The figure shows three views and two pictorial views of one solid part (mm, origin at its lowest corner). Answer the questions. A direction names the side the tool comes from. Give positions to 0.01 mm unless a question says otherwise; leave off trailing zeros. Loops run counter-clockwise (first coordinate to the right, second up) from the corner with the lowest first, then second, coordinate; pieces in that order, holes last. Notation, with made-up numbers: M 26.25,-0.5 L 69.25,-0.5 A20 cw 69.25,28.5 Z; hole C 27.5,-7.75 d9. An arc over 180 degrees is marked long. Write item = value, one per line. Start each with the question number.
1. Section B-B on z = 114.3 is taken. Determine the outline of the cut face in (x, y) (1 decimal).
2. Flat-ended cylindrical pins translate along their axes: pin 1 Ø10 at (x, y) = (28, 11.5) entering from +Z; pin 2 Ø10.5 at (y, z) = (12.5, 109.5) entering from +X (3 decimals); pin 3 Ø17.5 at (x, z) = (20.5, 104.5) entering from +Y (3 decimals). Find the tip coordinate at first contact, or state that the pin passes through.
3. Section D-D on x = 24 is taken. Determine the outline of the cut face in (y, z) (1 decimal).
4. Consider L1, parallel to Z at x = 2, y = 19; L2, parallel to Y at x = 2.45, z = 38.1; L3, parallel to Y at x = 23, z = 145 (1 decimal). Determine where each line is inside the solid, lowest interval first. Write a range as [from, to].
5. Section C-C on z = 57 is taken. Determine the outline of the cut face in (x, y) (1 decimal).
6. For the marked faces 1 and 2, determine the directions among +Z, -Z, +X, -X, +Y, -Y from which every point of the face is accessible in a straight line to the end or side of a thin tool.
7. Section A-A on y = 19.05 is taken. Determine the outline of the cut face in (x, z) (1 decimal), plus the area to 3 significant figures.
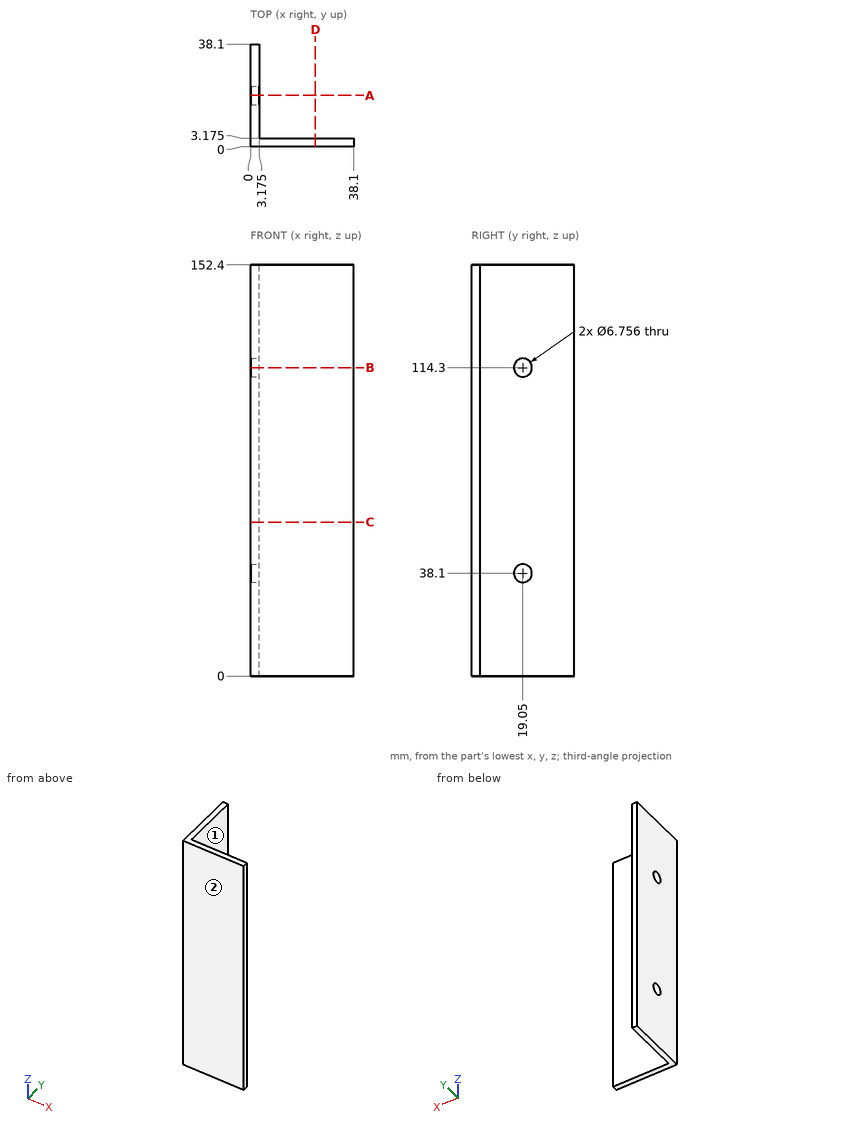
Verdict:
q1.outline = M 0,0 L 38.1,0 L 38.1,3.2 L 3.2,3.2 L 3.2,15.7 L 0,15.7 Z; M 0,22.4 L 3.2,22.4 L 3.2,38.1 L 0,38.1 Z
q2.pin_1 = through
q2.pin_2 = 3.175
q2.pin_3 = 3.175
q3.outline = M 0,0 L 3.2,0 L 3.2,152.4 L 0,152.4 Z
q4.L1 = [0, 34.72], [41.48, 110.92], [117.68, 152.4]
q4.L2 = [0, 15.67], [22.43, 38.1]
q4.L3 = [0, 3.2]
q5.outline = M 0,0 L 38.1,0 L 38.1,3.2 L 3.2,3.2 L 3.2,38.1 L 0,38.1 Z
q6.face_1 = +Z, -Z, +X, +Y
q6.face_2 = +Z, -Z, +X, -X, -Y
q7.outline = M 0,0 L 3.2,0 L 3.2,34.7 L 0,34.7 Z; M 0,41.5 L 3.2,41.5 L 3.2,110.9 L 0,110.9 Z; M 0,117.7 L 3.2,117.7 L 3.2,152.4 L 0,152.4 Z
q7.area = 441 mm2
